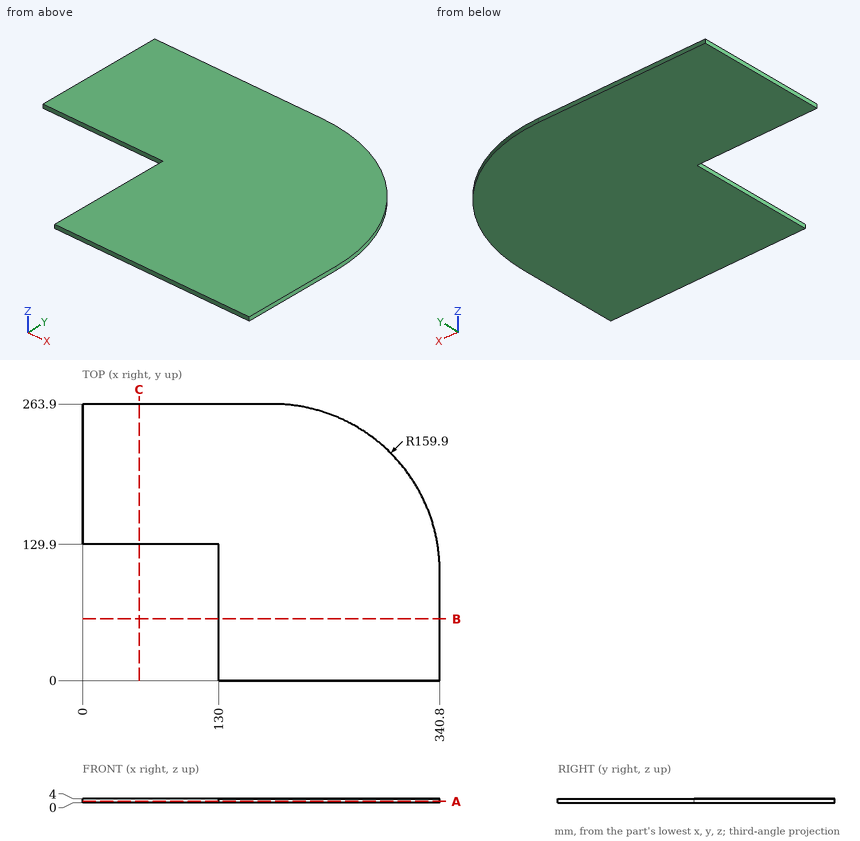
Could you check a few things on this drawing? It's one solid part, dimensions in mm from its lowest x, y, z. Coordinates: 2 decimals unless noted, no trailing zeros. Order: outer loops, then holes, each group sorted by start corner. A loop starts at its lowest first (then second) coordinate and runs counter-clockwise, first axis right, second up.
1) Imagine slicing it at A-A on z = 1.5. List the corners of the cut face in (x, y) for me, and give its area (3 significant figures).
2) I need wall thicknesses on line 1 (Y direction, x = 44, z = 2.5); line 2 (X direction, y = 22, z = 3.15); line 3 (Y direction, x = 255, z = 2.2). Which ranges of each line are inside material? Lowest first, please.
3) Imagine slicing it at B-B on y = 59. List the corners of the cut face in (x, z) for me.
4) Will these pins go through, and if not, where does the flat tip stop? pin 1 (2 mm diameter, centred on x = 271, z = 3.5, fed in from +Y) (3 decimals); pin 2 (1 mm diameter, centred on x = 91.5, z = 1.5, fed in from -Y).
5) Imagine slicing it at C-C on x = 54. List the corners of the cut face in (y, z) for me.
Response values:
1. outline: (0, 129.9) - (130, 129.9) - (130, 0) - (340.8, 0) - (340.8, 104) arc R159.9 ccw to (180.9, 263.9) - (0, 263.9) - close
1. area: 67,600 mm2
2. line 1: y = 129.9 to 263.9
2. line 2: x = 130 to 340.8
2. line 3: y = 0 to 245.69
3. outline: (130, 0) - (340.8, 0) - (340.8, 4) - (130, 4) - close
4. pin 1: stops at y = 236.775
4. pin 2: stops at y = 129.9
5. outline: (129.9, 0) - (263.9, 0) - (263.9, 4) - (129.9, 4) - close
